```python
from build123d import *

# Parameters (mm, degrees)
SKETCH1_R           = 2.5
BOSS_EXTRUDE1_DEPTH = 4


with BuildPart() as part:
    # Sketch1 → Boss-Extrude1 (new body)
    with BuildSketch(Plane(origin=(0, 0, 0), x_dir=(1, 0, 0), z_dir=(0, 1, 0))):
        with BuildLine():
            Line((-50, 0), (-50, -27))
            ThreePointArc((-50, -27), (-49.121320344, -29.121320344), (-47, -30))
            Line((-47, -30), (-33, -30))
            ThreePointArc((-33, -30), (-30.878679656, -29.121320344), (-30, -27))
            Line((-30, -27), (-30, -14.142135624))
            Line((-30, -14.142135624), (-30, 0))
            ThreePointArc((-30, 0), (-21.213203436, 21.213203436), (0, 30))
            Line((0, 30), (14.142135624, 30))
            Line((14.142135624, 30), (27, 30))
            ThreePointArc((27, 30), (29.121320344, 30.878679656), (30, 33))
            Line((30, 33), (30, 47))
            ThreePointArc((30, 47), (29.121320344, 49.121320344), (27, 50))
            Line((27, 50), (0, 50))
            ThreePointArc((0, 50), (-35.355339059, 35.355339059), (-50, 0))
        make_face()
        with Locations(Location((-40, -10, 0), (0, 0, 270))):
            Circle(SKETCH1_R, mode=Mode.SUBTRACT)
        with Locations(Location((-40, -25, 0), (0, 0, 270))):
            Circle(SKETCH1_R, mode=Mode.SUBTRACT)
        with Locations(Location((10, 40, 0), (0, 0, 270))):
            Circle(SKETCH1_R, mode=Mode.SUBTRACT)
        with Locations(Location((25, 40, 0), (0, 0, 270))):
            Circle(SKETCH1_R, mode=Mode.SUBTRACT)
    extrude(amount=BOSS_EXTRUDE1_DEPTH)


solid = part.part
```
For this review, take the finished solid that the model builds, in its own axes (mm). A direction names the side the tool comes from. Coordinates: 2 decimals unless noted, no trailing zeros. Order: outer loops, then holes, each group sorted by start corner. A loop starts at its lowest first (then second) coordinate and runs counter-clockwise, first axis right, second up. Notation, with made-up numbers: (42.25, 36.25) - (72.25, 36.25) arc R22 cw to (72.25, 68.25) - close; hole circle Ø1 at (-18, 70.25). An arc over 180 degrees is marked (long way). Answer as a JSON object with one key per item and string values. Group by question number.
1. We need section C-C on x = 25. State the section outline as (y, z) points, then the cut area to 3 significant figures.
2. The part is to be moulded in two halves that separate along X. For faces 3 (the flat face through (-40, 2, 30)), 4 (the cylindrical face through (27.11, 1.97, -38.66)), 5 (the cylindrical face through (-30.9, 1.97, 29.14)), say which applies: pulls with the +X half, pulls with the -X half, needs draft (parallel to the pull), parting line crosses it, or undercut.
3. We need section B-B on z = -40. State the section outline as (x, y) points, then the cut area to 3 significant figures.
4. Clearance check with flat-ended pins moving along their axes: P1, Ø2, axis at x = 17, y = 1.5, coming from the +Z side; P2, Ø2, axis at y = 1.5, z = 17.5, coming from the +X side; P3, Ø4.5, axis at x = 10, z = -40, coming from the +Y side; P4, Ø1.5, axis at y = 1, z = -37.5, coming from the -X side. State where each tip first meets the part, or that it passes through.
5. We need section A-A on x = -40. State the section outline as (y, z) points.
6. For faces 1 (the flat face through (13, 2, -30)), 2 (the cylindrical face through (-49.14, 1.97, 29.1)), list the 3-axis set-ups (+Z, -Z, +X, -X, +Y, -Y) from which the entire face can be reached by the end or side of a thin tool; tool diameter is ignored.
7. For probe 1 along X at (y, z) = (3.15, -40); probe 2 along X at (y, z) = (1.85, 10); probe 3 along Z at (x, y) = (-39, 1.3), list the stretches that pass through material, from the lowest coordinate up.
8. We need section D-D on y = 2. State the section outline as (x, z) points.
Final values:
{
 "1": {"outline": "(0, -50) - (4, -50) - (4, -42.5) - (0, -42.5) - close; (0, -37.5) - (4, -37.5) - (4, -30) - (0, -30) - close", "area": "60.0 mm²"},
 "2": {"face 3": "needs draft", "face 4": "undercut", "face 5": "pulls with the +X half"},
 "3": {"outline": "(-30, 0) - (7.5, 0) - (7.5, 4) - (-30, 4) - close; (12.5, 0) - (22.5, 0) - (22.5, 4) - (12.5, 4) - close; (27.5, 0) - (30, 0) - (30, 4) - (27.5, 4) - close", "area": "200 mm²"},
 "4": {"P1": "z = -30", "P2": "x = -30", "P3": "through", "P4": "x = -33.9"},
 "5": {"outline": "(0, -30) - (4, -30) - (4, 7.5) - (0, 7.5) - close; (0, 12.5) - (4, 12.5) - (4, 22.5) - (0, 22.5) - close; (0, 27.5) - (4, 27.5) - (4, 30) - (0, 30) - close"},
 "6": {"face 1": "+Z, +X, +Y, -Y", "face 2": "+Z, -X, +Y, -Y"},
 "7": {"probe 1": "-30 to 7.5, 12.5 to 22.5, 27.5 to 30", "probe 2": "-50 to -42.5, -37.5 to -30", "probe 3": "-31.29 to 7.71, 12.29 to 22.71, 27.29 to 30"},
 "8": {"outline": "(-50, 0) arc R50 ccw to (0, -50) - (27, -50) arc R3 ccw to (30, -47) - (30, -33) arc R3 ccw to (27, -30) - (0, -30) arc R30 cw to (-30, 0) - (-30, 27) arc R3 ccw to (-33, 30) - (-47, 30) arc R3 ccw to (-50, 27) - close; hole circle Ø5 at (-40, 10); hole circle Ø5 at (-40, 25); hole circle Ø5 at (10, -40); hole circle Ø5 at (25, -40)"}
}
